Can you work these out from the model? Positions are in its coordinate system, mm. A direction names the side the tool comes from. Coordinates: 2 decimals unless noted, no trailing zeros. Order: outer loops, then holes, each group sorted by start corner. A loop starts at its lowest first (then second) coordinate and runs counter-clockwise, first axis right, second up. Notation, with made-up numbers: M -2.75,52.25 L 2.25,52.25 A6 cw 2.25,60.25 Z; hole C -11.5,52 d9. An arc over 180 degrees is marked long. Answer as CSV lines item,"result". Start each with the question number.
1. On a 3-axis mill with a long thin cutter (end or side, diameter ignored), from which of +Z, -Z, +X, -X, +Y, -Y can I reach the whole of each face in a straight line? I mean faces 1 (the face through (-150, 1.27, -13)), 2 (the face through (-304.8, 1, -13)), 3 (the face through (-150, 7, -24.13)). Say none if no direction works.
2. I need wall thicknesses on line 1 along X through (y, z) = (0.75, -12.7) (3 decimals); line 2 along Z through (x, y) = (-83.5, 7); line 3 along Z through (x, y) = (-285.75, 0.9) (3 decimals). Which ranges of each line are inside material? Lowest first, please. Write a range as from..to.
3. If we section it at C-C (x = -19.05): List the corners of the cut face in (y, z) for me (3 decimals).
4. If we section it at A-A (z = -12.7): List the corners of the cut face in (x, y) for me (3 decimals), plus the area to 3 significant figures.
5. If we mould it in two halves opening along Z, with no side actions, what happens to faces 4 (the face through (-150, 5, -25.4)), 5 (the face through (-150, 0, -13)), 6 (the face through (-15.95, 0.64, -12.01)), 7 (the face through (-150, 7, -1.27))? For each: released by +Z, released by -Z, zero draft, split by the parting line, or undercut.
6. If we section it at D-D (x = -95.5): List the corners of the cut face in (y, z) for me, plus the area to 3 significant figures.
7. Will these pins go through, and if not, where does the flat tip stop? pin 1 (6 mm diameter, centred on x = -183.5, z = -16.5, fed in from +Y); pin 2 (5 mm diameter, centred on x = -41.5, z = -21, fed in from +Y).
8. If we section it at B-B (y = 7): List the corners of the cut face in (x, z) for me.
```python
from build123d import *

# Parameters (mm, degrees)
BOSS_EXTRUDE1_DEPTH = 304.8
SKETCH2_R           = 3.175
CUT_EXTRUDE2_DEPTH  = 306.985673031


with BuildPart() as part:
    # Sketch1 → Boss-Extrude1 (new body)
    with BuildSketch(Plane(origin=(0, 0, 0), x_dir=(0, 0, -1), z_dir=(1, 0, 0))):
        Polygon((0, 0), (25.4, 0), (25.4, 10.16), (24.13, 10.16), (24.13, 3.81), (22.224108836, 3.81), (22.224108836, 2.54), (24.13, 2.54), (24.13, 1.27), (1.27, 1.27), (1.27, 2.54), (3.175891164, 2.54), (3.175891164, 3.81), (1.27, 3.81), (1.27, 10.16), (0, 10.16), align=None)
    extrude(amount=-BOSS_EXTRUDE1_DEPTH)

    # Sketch2 → Cut-Extrude2 (cut, through all)
    with BuildSketch(Plane(origin=(0, 1.27, 0), x_dir=(1, 0, 0), z_dir=(0, 1, 0))):
        with Locations(Location((-285.75, 12.7, 0), (0, 0, 270))):
            Circle(SKETCH2_R)
        with Locations(Location((-19.05, 12.7, 0), (0, 0, 90))):
            Circle(SKETCH2_R)
    extrude(amount=-CUT_EXTRUDE2_DEPTH, mode=Mode.SUBTRACT)


solid = part.part
```
Solved:
1,face 1,"+X, -X"
1,face 2,"+Z, -Z, -X, +Y, -Y"
1,face 3,"+X, -X, +Y"
2,line 1,"-304.8..-288.925, -282.575..-22.225, -15.875..0"
2,line 2,"-25.4..-24.13, -1.27..0"
2,line 3,"-25.4..-15.875, -9.525..0"
3,outline,"M 0,-25.4 L 10.16,-25.4 L 10.16,-24.13 L 3.81,-24.13 L 3.81,-22.224 L 2.54,-22.224 L 2.54,-24.13 L 1.27,-24.13 L 1.27,-15.875 L 0,-15.875 Z; M 0,-9.525 L 1.27,-9.525 L 1.27,-1.27 L 2.54,-1.27 L 2.54,-3.176 L 3.81,-3.176 L 3.81,-1.27 L 10.16,-1.27 L 10.16,0 L 0,0 Z"
4,outline,"M -304.8,0 L -288.925,0 L -288.925,1.27 L -304.8,1.27 Z; M -282.575,0 L -22.225,0 L -22.225,1.27 L -282.575,1.27 Z; M -15.875,0 L 0,0 L 0,1.27 L -15.875,1.27 Z"
4,area,"371 mm²"
5,face 4,"released by -Z"
5,face 5,"zero draft"
5,face 6,"undercut"
5,face 7,"undercut"
6,outline,"M 0,-25.4 L 10.16,-25.4 L 10.16,-24.13 L 3.81,-24.13 L 3.81,-22.22 L 2.54,-22.22 L 2.54,-24.13 L 1.27,-24.13 L 1.27,-1.27 L 2.54,-1.27 L 2.54,-3.18 L 3.81,-3.18 L 3.81,-1.27 L 10.16,-1.27 L 10.16,0 L 0,0 Z"
6,area,"59.7 mm²"
7,pin 1,"y = 1.27"
7,pin 2,"y = 3.81"
8,outline,"M -304.8,-25.4 L 0,-25.4 L 0,-24.13 L -304.8,-24.13 Z; M -304.8,-1.27 L 0,-1.27 L 0,0 L -304.8,0 Z"
